The model under review builds one solid part; all positions refer to its coordinate system, in mm. A direction names the side the tool comes from. Round coordinates to 2 decimals unless told otherwise and drop trailing zeros. Order: outer loops, then holes, each group sorted by start corner. A loop starts at its lowest first (then second) coordinate and runs counter-clockwise, first axis right, second up. Notation, with made-up numbers: M 31.25,88.5 L 62.25,88.5 A13 ccw 62.25,99.5 Z; hole C 1,2.25 d4. An arc over 180 degrees is marked long. Answer as a JSON object with one key per item and string values. Group by question number.
1. Add section D-D on x = 5. State the section outline as (y, z) points, and give its area (3 significant figures).
2. Add section B-B on z = -3.5. State the section outline as (x, y) points.
3. Add section A-A on y = 0. State the section outline as (x, z) points, and give its area (3 significant figures).
4. Clearance check with flat-ended pins moving along their axes: P1, Ø8, axis at x = -12, y = -4, coming from the +Z side; P2, Ø8, axis at x = -10.5, y = -1, coming from the -Z side; P3, Ø1, axis at x = 15, y = 3.5, coming from the +Z side. State where each tip first meets the part, or that it passes through.
5. Add section C-C on y = 4. State the section outline as (x, z) points, and give its area (3 significant figures).
6. Machinability: for faces 1 (the face through (-12, 0, -20.187)), 2 (the face through (-12, 0, -25.267)), 3 (the face through (1.211, -5, -10)), which of the approach directions +Z, -Z, +X, -X, +Y, -Y give a long, thin tool a straight path to every point of the face, cutting with its end or side? Answer none if there is none.
7. To check wall thickness, follow probe 1 along X at (y, z) = (5.5, -23); probe 2 along Z at (x, y) = (46, -2); probe 3 along X at (y, z) = (4.25, 11). State the ranges of each line that lie inside material, in increasing order. Write a range as [from, to].
8. Mouldability with a two-part tool opening along Z and no side actions: class faces 4 (the face through (-2.758, 0, 15)), 5 (the face through (29, 0, -41.258)), 6 (the face through (-2.758, 0, -7)) as released by +Z, released by -Z, zero draft, split by the parting line, or undercut.
```python
from build123d import *

# Parameters (mm, degrees)
BOSS_EXTRUDE1_DEPTH = 7.9375
SKETCH3_R           = 5.207
CUT_EXTRUDE1_DEPTH  = 3.96875
SKETCH4_R           = 1.2065
BOSS_EXTRUDE2_DEPTH = 8.89
SKETCH5_W           = 5.08
SKETCH5_H           = 15.875
BOSS_EXTRUDE3_DEPTH = 18.288


with BuildPart() as part:
    # Sketch1 → Boss-Extrude1 (new, symmetric)
    with BuildSketch(Plane(origin=(0, 0, 0), x_dir=(1, 0, 0), z_dir=(0, 1, 0))):
        Polygon((-2.757708096, -19.86108723), (1.211041904, -19.86108723), (1.211041904, 41.25766277), (58.361041904, 41.25766277), (58.361041904, 45.22641277), (6.27967861, 45.22641277), (-2.757708096, 45.22641277), align=None)
    extrude(amount=BOSS_EXTRUDE1_DEPTH, both=True)

    # Sketch3 → Cut-Extrude1 (cut)
    with BuildSketch(Plane.ZY.offset(2.757708096)):
        with Locations((-12.566559842, 0)):
            Circle(SKETCH3_R)
    extrude(amount=-CUT_EXTRUDE1_DEPTH, mode=Mode.SUBTRACT)

    # Sketch4 → Boss-Extrude2 (add)
    with BuildSketch(Plane(origin=(0, 0, -45.22641277), x_dir=(-1, 0, 0), z_dir=(0, 0, -1))):
        with Locations(Location((-22.007291904, 0, 0), (0, 0, 180))):
            Circle(SKETCH4_R)
    extrude(amount=BOSS_EXTRUDE2_DEPTH)

    # Sketch5 → Boss-Extrude3 (add)
    with BuildSketch(Plane.ZY.offset(2.757708096)):
        with Locations((-22.726559842, 0)):
            Rectangle(SKETCH5_W, SKETCH5_H)
        with Locations((8.388440158, 0)):
            Rectangle(SKETCH5_W, SKETCH5_H)
    extrude(amount=BOSS_EXTRUDE3_DEPTH)


solid = part.part
```
Recorded:
{
 "1": {"outline": "M -7.94,-45.23 L 7.94,-45.23 L 7.94,-41.26 L -7.94,-41.26 Z", "area": "63.0 mm²"},
 "2": {"outline": "M -2.76,-7.94 L 1.21,-7.94 L 1.21,7.94 L -2.76,7.94 Z"},
 "3": {"outline": "M -21.05,-25.27 L -2.76,-25.27 L -2.76,-45.23 L 20.8,-45.23 L 20.8,-54.12 L 23.21,-54.12 L 23.21,-45.23 L 58.36,-45.23 L 58.36,-41.26 L 1.21,-41.26 L 1.21,-17.77 L -2.76,-17.77 L -2.76,-20.19 L -21.05,-20.19 Z; M -21.05,5.85 L -2.76,5.85 L -2.76,-7.36 L 1.21,-7.36 L 1.21,19.86 L -2.76,19.86 L -2.76,10.93 L -21.05,10.93 Z", "area": "651 mm²"},
 "4": {"P1": "stops at z = 10.93", "P2": "stops at z = -25.27", "P3": "stops at z = -41.26"},
 "5": {"outline": "M -21.05,-25.27 L -2.76,-25.27 L -2.76,-45.23 L 58.36,-45.23 L 58.36,-41.26 L 1.21,-41.26 L 1.21,-15.9 L -2.76,-15.9 L -2.76,-20.19 L -21.05,-20.19 Z; M -21.05,5.85 L -2.76,5.85 L -2.76,-9.23 L 1.21,-9.23 L 1.21,19.86 L -2.76,19.86 L -2.76,10.93 L -21.05,10.93 Z", "area": "644 mm²"},
 "6": {"face 1": "-X, +Y, -Y", "face 2": "-Z, -X, +Y, -Y", "face 3": "+Z, +X, +Y, -Y"},
 "7": {"probe 1": "x = [-21.05, 1.21]", "probe 2": "z = [-45.23, -41.26]", "probe 3": "x = [-2.76, 1.21]"},
 "8": {"face 4": "zero draft", "face 5": "released by +Z", "face 6": "undercut"}
}
